Geometry check sheet. Reference: the model listing, model coordinates, mm. Face numbers are marked on the shaded views. A direction names the side the tool comes from. Round coordinates to 2 decimals unless told otherwise and drop trailing zeros. Write each loop counter-clockwise with the first axis right and the second up, starting at its lowest first coordinate (ties: lowest second). Pieces come first, ordered by that corner, then holes. Notation, with made-up numbers: (15.5, 23) - (30.5, 23) arc R28 cw to (30.5, 59) - close; hole circle Ø2 at (49, 54). An arc over 180 degrees is marked (long way). Return JSON: item names as keys, results as strings.
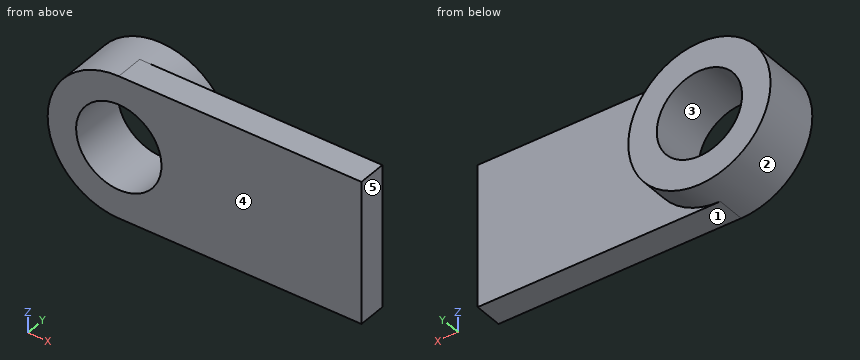
```python
from build123d import *

# Parameters (mm, degrees)
SKETCH1_R           = 15.875
SKETCH1_R_2         = 9.525
BOSS_EXTRUDE1_DEPTH = 12.7
BOSS_EXTRUDE2_DEPTH = 6.35


with BuildPart() as part:
    # Sketch1 → Boss-Extrude1 (new body)
    with BuildSketch(Plane(origin=(0, 0, 0), x_dir=(1, 0, 0), z_dir=(0, 1, 0))):
        with Locations(Location((0, 0, 0), (0, 0, 270))):
            Circle(SKETCH1_R)
        with Locations(Location((0, 0, 0), (0, 0, 270))):
            Circle(SKETCH1_R_2, mode=Mode.SUBTRACT)
    extrude(amount=BOSS_EXTRUDE1_DEPTH)

    # Sketch1_6 → Boss-Extrude2 (add)
    with BuildSketch(Plane(origin=(0, 0, 0), x_dir=(1, 0, 0), z_dir=(0, 1, 0))):
        with BuildLine():
            ThreePointArc((15.875, 0), (11.225320151, -11.225320151), (0, -15.875))
            Line((0, -15.875), (54.154575014, -15.875))
            Line((54.154575014, -15.875), (54.154575014, 15.875))
            Line((54.154575014, 15.875), (0, 15.875))
            ThreePointArc((0, 15.875), (11.225320151, 11.225320151), (15.875, 0))
        make_face()
    extrude(amount=BOSS_EXTRUDE2_DEPTH)


solid = part.part
```
(1) Material ranges on line 1 along X through (y, z) = (9.25, 0) (3 decimals); line 2 along X through (y, z) = (5.5, 0) (3 decimals); line 3 along Z through (x, y) = (-7.5, 6.25), recorded low to high. Write a range as [from, to].
Response values:
{"line 1": "x = [-15.875, -9.525], [9.525, 15.875]", "line 2": "x = [-15.875, -9.525], [9.525, 54.155]", "line 3": "z = [-13.99, -5.87], [5.87, 13.99]"}
(2) Section check A-A, the plane z = 0. Enter the section's corners in (x, y) (3 decimals).
Response values:
{"outline": "(-15.875, 0) - (-9.525, 0) - (-9.525, 12.7) - (-15.875, 12.7) - close; (9.525, 0) - (54.155, 0) - (54.155, 6.35) - (15.875, 6.35) - (15.875, 12.7) - (9.525, 12.7) - close"}
(3) Section check C-C, the plane x = -6. Enter the section's corners in (y, z).
Response values:
{"outline": "(0, -14.7) - (12.7, -14.7) - (12.7, -7.4) - (0, -7.4) - close; (0, 7.4) - (12.7, 7.4) - (12.7, 14.7) - (0, 14.7) - close"}
(4) Access from +Z, -Z, +X, -X, +Y, -Y to the whole of each face (thin tool, end or side, straight path). Record for the marked faces 1 and 2.
Response values:
{"face 1": "-Z, +X, -X, +Y, -Y", "face 2": "+Y"}
(5) Release check for a two-part mould opening along X. For the marked faces 3, 4 and 5 record: pulls with the +X half, pulls with the -X half, needs draft (parallel to the pull), parting line crosses it, or undercut.
Response values:
{"face 3": "undercut", "face 4": "needs draft", "face 5": "pulls with the +X half"}
(6) Section check B-B, the plane y = 1.5. Enter the section's corners in (x, z) (3 decimals).
Response values:
{"outline": "(0, -15.875) - (54.155, -15.875) - (54.155, 15.875) - (0, 15.875) arc R15.875 ccw to start; hole circle Ø19.05 at (0, 0)"}
(7) Gauge pin test, flat ends, axial feed: pin 1 (6 mm diameter, centred on x = 8.5, y = 9.5, fed in from +Z); pin 2 (15 mm diameter, centred on x = 0, z = 0, fed in from -Y); pin 3 (4 mm diameter, centred on y = 11.5, z = -10, fed in from -X); pin 4 (2 mm diameter, centred on y = 9.5, z = 3, fed in from -X). Record the tip position at first contact, or that the pin passes through.
Response values:
{"pin 1": "stops at z = 14.89", "pin 2": "passes through", "pin 3": "stops at x = -13.71", "pin 4": "stops at x = -15.75"}
(8) Section check D-D, the plane x = 12. Enter the section's corners in (y, z) (3 decimals), plus the area to 3 significant figures.
Response values:
{"outline": "(0, -15.875) - (6.35, -15.875) - (6.35, -10.393) - (12.7, -10.393) - (12.7, 10.393) - (6.35, 10.393) - (6.35, 15.875) - (0, 15.875) - close", "area": "334 mm^2"}
